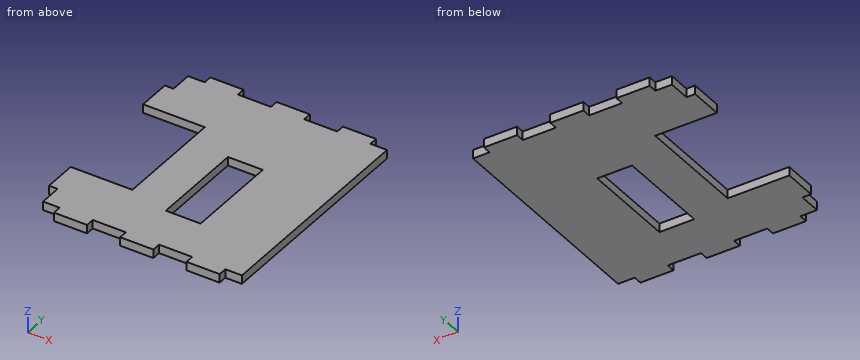
from build123d import *

# Parameters (mm, degrees)
SKETCH1_W           = 114.3
SKETCH1_H           = 127.2286
BOSS_EXTRUDE1_DEPTH = 2.48046875
SKETCH3_W           = 19.05
SKETCH3_H           = 4.9609375
BOSS_EXTRUDE2_DEPTH = 4.9609375
SKETCH5_W           = 19.05
SKETCH5_H           = 4.9609375
BOSS_EXTRUDE3_DEPTH = 4.9784
SKETCH7_W           = 4.9609375
SKETCH7_H           = 63.5
CUT_EXTRUDE1_DEPTH  = 30.48
SKETCH6_W           = 4.9609375
SKETCH6_H           = 19.05
BOSS_EXTRUDE4_DEPTH = 4.9609375
CAVITY1_START       = -3.0309375
CAVITY1_2_OUTLINE_W = 41
CAVITY1_2_OUTLINE_H = 4.9609375
CAVITY1_2_DEPTH     = 19
CAVITY1_START_2     = -2.3309375
CAVITY1_3_DEPTH     = 17.6
CAVITY1_START_3     = -3
CAVITY1_4_DEPTH     = 6
CAVITY1_START_4     = 0.91953125
CAVITY1_6_OUTLINE_R = 3
CAVITY1_6_DEPTH     = 1.5609375
SKETCH9_W           = 20
SKETCH9_H           = 54.483
CUT_EXTRUDE2_DEPTH  = 93.827315363


with BuildPart() as part:
    # Sketch1 → Boss-Extrude1 (new, symmetric)
    with BuildSketch(Plane.XY):
        Rectangle(SKETCH1_W, SKETCH1_H)
    extrude(amount=BOSS_EXTRUDE1_DEPTH, both=True)

    # Sketch3 → Boss-Extrude2 (add)
    with BuildSketch(Plane(origin=(0, 63.6143, 0), x_dir=(1, 0, 0), z_dir=(0, 1, 0))):
        with Locations((38.1, 0)):
            Rectangle(SKETCH3_W, SKETCH3_H)
        Rectangle(SKETCH3_W, SKETCH3_H)
        with Locations((-38.1, 0)):
            Rectangle(SKETCH3_W, SKETCH3_H)
    extrude(amount=BOSS_EXTRUDE2_DEPTH)

    # Sketch5 → Boss-Extrude3 (add)
    with BuildSketch(Plane.XZ.offset(63.6143)):
        Rectangle(SKETCH5_W, SKETCH5_H)
        with Locations((38.1, 0)):
            Rectangle(SKETCH5_W, SKETCH5_H)
        with Locations((-38.1, 0)):
            Rectangle(SKETCH5_W, SKETCH5_H)
    extrude(amount=BOSS_EXTRUDE3_DEPTH)

    # Sketch7 → Cut-Extrude1 (cut)
    with BuildSketch(Plane.ZY.offset(57.15)):
        Rectangle(SKETCH7_W, SKETCH7_H)
    extrude(amount=-CUT_EXTRUDE1_DEPTH, mode=Mode.SUBTRACT)

    # Sketch6 → Boss-Extrude4 (add)
    with BuildSketch(Plane.ZY.offset(57.15)):
        with Locations((0, 41.275)):
            Rectangle(SKETCH6_W, SKETCH6_H)
        with Locations((0, -41.275)):
            Rectangle(SKETCH6_W, SKETCH6_H)
    extrude(amount=BOSS_EXTRUDE4_DEPTH)

    # Cavity1: read off the stored shape, not the designer's step
    # Cavity1 outline → Cavity1 (revolve, cut)
    with BuildSketch(Plane(origin=(15.2690625, 0, -2.53046875), x_dir=(1, 0, 0), z_dir=(0, 0, 1))):
        with BuildLine():
            ThreePointArc((0.05, -31.0547625), (0.064644661, -31.019407161), (0.1, -31.0047625))
            Line((0.1, -31.0047625), (0.1, 9.9952375))
            ThreePointArc((0.1, 9.9952375), (0.064644661, 10.009882161), (0.05, 10.0452375))
            Line((0.05, 10.0452375), (0.05, -31.0547625))
        make_face()
    revolve(axis=Axis((15.2690625, 0, -2.53046875), (0, 1, 0)), mode=Mode.SUBTRACT)

    # Cavity1 2 outline → Cavity1 2 (cut)
    with BuildSketch(Plane.YZ.offset(CAVITY1_START)):
        with Locations((-10.5047625, 0)):
            Rectangle(CAVITY1_2_OUTLINE_W, CAVITY1_2_OUTLINE_H)
    extrude(amount=CAVITY1_2_DEPTH, mode=Mode.SUBTRACT)

    # Cavity1 3 outline → Cavity1 3 (cut)
    with BuildSketch(Plane.YZ.offset(CAVITY1_START_2)):
        with BuildLine():
            ThreePointArc((-31.0047625, -2.43046875), (-31.019407161, -2.465824089), (-31.0547625, -2.48046875))
            Line((-31.0547625, -2.48046875), (-31.0047625, -2.48046875))
            Line((-31.0047625, -2.48046875), (-31.0047625, -2.43046875))
        make_face()
        with BuildLine():
            Line((9.9952375, -2.43046875), (9.9952375, -2.48046875))
            Line((9.9952375, -2.48046875), (10.0452375, -2.48046875))
            ThreePointArc((10.0452375, -2.48046875), (10.009882161, -2.465824089), (9.9952375, -2.43046875))
        make_face()
    extrude(amount=CAVITY1_3_DEPTH, mode=Mode.SUBTRACT)

    # Cavity1 4 outline → Cavity1 4 (cut)
    with BuildSketch(Plane.XY.offset(CAVITY1_START_3)):
        with BuildLine():
            ThreePointArc((15.9690625, -31.0047625), (16.322615891, -30.858315891), (16.4690625, -30.5047625))
            Line((16.4690625, -30.5047625), (16.4690625, 9.4952375))
            ThreePointArc((16.4690625, 9.4952375), (16.322615891, 9.848790891), (15.9690625, 9.9952375))
            Line((15.9690625, 9.9952375), (15.9690625, -31.0047625))
        make_face()
        with BuildLine():
            ThreePointArc((-3.0309375, 9.9952375), (-3.384490891, 9.848790891), (-3.5309375, 9.4952375))
            Line((-3.5309375, 9.4952375), (-3.5309375, -30.5047625))
            ThreePointArc((-3.5309375, -30.5047625), (-3.384490891, -30.858315891), (-3.0309375, -31.0047625))
            Line((-3.0309375, -31.0047625), (-3.0309375, 9.9952375))
        make_face()
    extrude(amount=CAVITY1_4_DEPTH, mode=Mode.SUBTRACT)

    # Cavity1 5 outline → Cavity1 5 (revolve, cut)
    with BuildSketch(Plane(origin=(-2.3309375, 0, -2.53046875), x_dir=(1, 0, 0), z_dir=(0, 0, 1))):
        with BuildLine():
            ThreePointArc((0.05, -31.0547625), (0.064644661, -31.019407161), (0.1, -31.0047625))
            Line((0.1, -31.0047625), (0.05, -31.0047625))
            Line((0.05, -31.0047625), (0.05, -31.0547625))
        make_face()
        with BuildLine():
            Line((0.05, 9.9952375), (0.1, 9.9952375))
            ThreePointArc((0.1, 9.9952375), (0.064644661, 10.009882161), (0.05, 10.0452375))
            Line((0.05, 10.0452375), (0.05, 9.9952375))
        make_face()
    revolve(axis=Axis((-2.3309375, 0, -2.53046875), (0, 1, 0)), mode=Mode.SUBTRACT)


with BuildPart() as body_2:
    # Cavity1 6 outline → Cavity1 6 (new body)
    with BuildSketch(Plane.XY.offset(CAVITY1_START_4)):
        with Locations((6.4690625, -0.0047625)):
            Circle(CAVITY1_6_OUTLINE_R)
    extrude(amount=CAVITY1_6_DEPTH)


with BuildPart() as cut_extrude2_tool:
    # Sketch9 → Cut-Extrude2 (new, through all)
    with BuildSketch(Plane(origin=(0, 0, -4.88046875), x_dir=(-1, 0, 0), z_dir=(0, 0, -1))):
        with Locations((-6.4690625, -10.5047625)):
            Rectangle(SKETCH9_W, SKETCH9_H)
    extrude(amount=-CUT_EXTRUDE2_DEPTH)


with BuildPart() as part_1:
    add(part.part)

    # Cut-Extrude2: cut by cut_extrude2_tool
    add(cut_extrude2_tool.part, mode=Mode.SUBTRACT)


with BuildPart() as body_2_1:
    add(body_2.part)

    # Cut-Extrude2: cut by cut_extrude2_tool
    add(cut_extrude2_tool.part, mode=Mode.SUBTRACT)


solid = part_1.part
Build history of the part. All positions in model axes, mm. Round coordinates to 2 decimals unless told otherwise and drop trailing zeros. Write each loop counter-clockwise with the first axis right and the second up, starting at its lowest first coordinate (ties: lowest second). Pieces come first, ordered by that corner, then holes. Notation, with made-up numbers: M 4,50 L 11,50 A23 cw 11,70 Z; hole C 44,11 d7. An arc over 180 degrees is marked long. Answer as a JSON object with one key per item and string values. Group by question number.
(1) Cut at C-C (x = -21). Give the cut face in (y, z), and give its area (3 significant figures).
(2) Cut at A-A (x = -39). Give the cut face in (y, z), and give its area (3 significant figures).
(3) Drill centre lines: L1, parallel to X at y = -23, z = -0.25; L2, parallel to Y at x = 16, z = -0.55; L3, parallel to Y at x = -32, z = 0.15. Where is each one in solid material? Low to high.
(4) Cut at B-B (y = -21). Give the cut face in (x, z).
(5) Flat gauge pins, fed straight in: pin 1 (2 mm diameter, centred on x = -49.5, z = 1, fed in from +Y); pin 2 (1.5 mm diameter, centred on y = -67, z = -1, fed in from -X) (3 decimals); pin 3 (1.5 mm diameter, centred on y = -57.5, z = -0.5, fed in from -X). Where does each tip first touch, or does it go through?
(6) Cut at D-D (y = 60.5). Give the cut face in (x, z), and give its area (3 significant figures).
Responses:
{
 "1": {"outline": "M -63.61,-2.48 L 63.61,-2.48 L 63.61,2.48 L -63.61,2.48 Z", "area": "631 mm2"},
 "2": {"outline": "M -68.59,-2.48 L -31.75,-2.48 L -31.75,2.48 L -68.59,2.48 Z; M 31.75,-2.48 L 68.58,-2.48 L 68.58,2.48 L 31.75,2.48 Z", "area": "365 mm2"},
 "3": {"L1": "x = -26.67 to -3.53, 16.47 to 57.15", "L2": "y = -63.61 to -37.75, 16.74 to 63.61", "L3": "y = -68.59 to -31.75, 31.75 to 68.58"},
 "4": {"outline": "M -26.67,-2.48 L -3.53,-2.48 L -3.53,2.48 L -26.67,2.48 Z; M 16.47,-2.48 L 57.15,-2.48 L 57.15,2.48 L 16.47,2.48 Z"},
 "5": {"pin 1": "stops at y = 63.61", "pin 2": "stops at x = -47.625", "pin 3": "stops at x = -57.15"},
 "6": {"outline": "M -57.15,-2.48 L 57.15,-2.48 L 57.15,2.48 L -57.15,2.48 Z", "area": "567 mm2"}
}
